Model file for the job. Use its own axes, mm. Face numbers are marked on the shaded views. A direction names the side the tool comes from. Round coordinates to 2 decimals unless told otherwise and drop trailing zeros. Loops run counter-clockwise (first coordinate to the right, second up) from the corner with the lowest first, then second, coordinate; pieces in that order, holes last. Notation, with made-up numbers: (30.5, 75.5) - (84.5, 75.5) arc R14 cw to (84.5, 95.5) - close; hole circle Ø6 at (69.25, 79). An arc over 180 degrees is marked (long way). Use one line per item in the form item = value.
from build123d import *


with BuildPart() as f2:
    # F2: sweep along a path in F1
    with BuildLine(Plane.YZ) as f2_path:
        Line((0, 0), (54.2271062732, 0))
        Line((54.2271062732, 0), (74.3272826076, -27.5529418141))
        Line((74.3272826076, -27.5529418141), (95.5489575863, -51.0973446071))
        Line((95.5489575863, -51.0973446071), (104.9186140299, -76.3795748353))
        Line((104.9186140299, -76.3795748353), (119.5624619722, -90.8030569553))
        Line((119.5624619722, -90.8030569553), (134.8015367985, -95.1338708401))
        Line((134.8015367985, -95.1338708401), (147.8405743837, -95.1338708401))
    # F0 (on Front) → F2 (sweep)
    with BuildSketch(Plane.XZ):
        with BuildLine():
            Line((-51.6746714711, 23.7191500306), (-51.6746714711, 0))
            ThreePointArc((-51.6746714711, 0), (-49.8239963657, -4.4809123505), (-45.350710686, -6.3499466107))
            Line((-45.350710686, -6.3499466107), (47.1804031889, -6.7293887862))
            ThreePointArc((47.1804031889, -6.7293887862), (51.089613293, -5.4037315626), (53.357891469, -1.9549339708))
            Line((53.357891469, -1.9549339708), (59.5256559013, 22.1268726525))
            ThreePointArc((59.5256559013, 22.1268726525), (58.3905238566, 27.5958286572), (53.374206836, 30.0523644478))
            Line((53.374206836, 30.0523644478), (51.2866688171, 30.0523644478))
            ThreePointArc((51.2866688171, 30.0523644478), (47.2485796403, 28.6030109154), (45.0538349714, 24.9165646999))
            Line((45.0538349714, 24.9165646999), (41.2004016239, 5.1357997479))
            ThreePointArc((41.2004016239, 5.1357997479), (39.005656955, 1.4493535324), (34.9675677782, 0))
            Line((34.9675677782, 0), (-31.172045563, 0))
            ThreePointArc((-31.172045563, 0), (-35.3717492022, 1.587123837), (-37.472098588, 5.5551214666))
            Line((-37.472098588, 5.5551214666), (-39.8641464341, 24.514028564))
            ThreePointArc((-39.8641464341, 24.514028564), (-41.8092828653, 28.3405352625), (-45.7444354651, 30.0552606822))
            ThreePointArc((-45.7444354651, 30.0552606822), (-49.9608337505, 28.0583319027), (-51.6746714711, 23.7191500306))
        make_face()
    sweep(path=f2_path.line, transition=Transition.RIGHT)


solid = f2.part
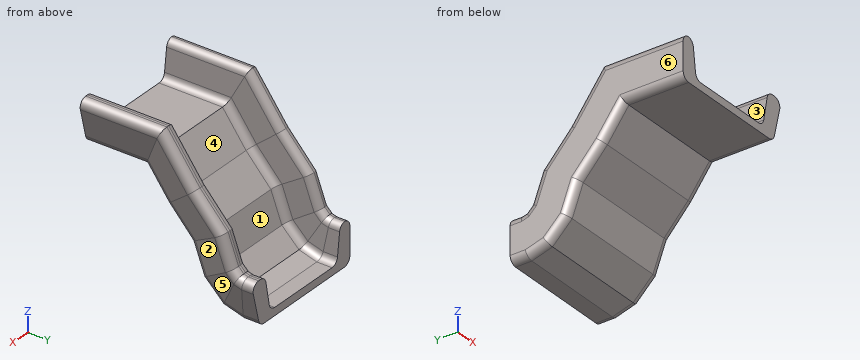
1. Cut at B-B, the plane x = -2.5. Give the cut face in (y, z).
Geometry check:
outline = (0, -6.53) - (50.91, -6.53) - (69.25, -31.67) - (89.86, -54.54) - (99.3, -80.01) - (116.17, -96.62) - (133.89, -101.66) - (147.84, -101.66) - (147.84, -95.13) - (134.8, -95.13) - (119.56, -90.8) - (104.92, -76.38) - (95.55, -51.1) - (74.33, -27.55) - (54.23, 0) - (0, 0) - close
2. Pull direction X, two halves, no side cores. Call the marked faces 4, 5 and 6: +X half, -X half, draft (parallel to the pull), parting line (faces both ways), or undercut.
Geometry check:
face_4 = undercut
face_5 = +X half
face_6 = -X half
3. Flat gauge pins, fed straight in: pin 1 (12 mm diameter, centred on x = -23.5, z = -79.5, fed in from +Y); pin 2 (3 mm diameter, centred on y = 74.5, z = 9, fed in from +X); pin 3 (6 mm diameter, centred on y = 50, z = -5.5, fed in from +X). Where does each tip first touch, or does it go through?
Geometry check:
pin_1 = 114.18
pin_2 = 59.7
pin_3 = 53.19
4. Wall check: probe 1 along X at (y, z) = (118.5, -78); probe 2 along X at (y, z) = (80.5, 0.5); probe 3 along Y at (x, z) = (8.5, -32). Give the ranges that are in metal, low to high.
Geometry check:
probe_1 = -51.67 to -37.83, 41.83 to 56
probe_2 = -51.67 to -39.49, 44.39 to 59.37
probe_3 = 69.49 to 78.34
5. Cut at C-C, the plane x = 17.5. Give the cut face in (y, z).
Geometry check:
outline = (0, -6.61) - (50.87, -6.61) - (69.19, -31.72) - (89.79, -54.58) - (99.23, -80.06) - (116.13, -96.7) - (133.88, -101.74) - (147.84, -101.74) - (147.84, -95.13) - (134.8, -95.13) - (119.56, -90.8) - (104.92, -76.38) - (95.55, -51.1) - (74.33, -27.55) - (54.23, 0) - (0, 0) - close
6. Tool access for the marked faces 1, 2 and 3: list every direction of +Z, -Z, +X, -X, +Y, -Y with a clear straight run to the whole face (end or side of a thin tool).
Geometry check:
face_1 = +Z, +Y
face_2 = -Z, +X, -Y
face_3 = +Z, +Y, -Y
7. Cut at A-A, the plane y = 18.5. Give the cut face in (x, z), plus the area to 3 significant figures.
Geometry check:
outline = (-51.67, 0) arc R6.35 ccw to (-45.35, -6.35) - (47.18, -6.73) arc R6.35 ccw to (53.36, -1.95) - (59.53, 22.13) arc R6.35 ccw to (53.37, 30.05) - (51.29, 30.05) arc R6.35 ccw to (45.05, 24.92) - (41.2, 5.14) arc R6.35 cw to (34.97, 0) - (-31.17, 0) arc R6.35 cw to (-37.47, 5.56) - (-39.86, 24.51) arc R6.35 ccw to (-45.74, 30.06) arc R6.35 ccw to (-51.67, 23.72) - close
area = 1,480 mm^2
